```python
from build123d import *

# Parameters (mm, degrees)
F1_DEPTH = 12.7
F2_R     = 15.24
F3_R     = 5.08
F6_DEPTH = 1.27
F9_DEPTH = 1.27


with BuildPart() as f1:
    # F0 (on Front) → F1 (new body)
    with BuildSketch(Plane.XZ):
        with BuildLine():
            ThreePointArc((41.717369, 0.82729), (26.878905, 42.014486), (0, 76.570086))
            ThreePointArc((0, 76.570086), (-26.878905, 42.014486), (-41.717369, 0.82729))
            Line((-41.717369, 0.82729), (-36.542559, 0.82729))
            ThreePointArc((-36.542559, 0.82729), (-23.349687, 37.863578), (0, 69.494744))
            ThreePointArc((0, 69.494744), (23.349687, 37.863578), (36.542559, 0.82729))
            Line((36.542559, 0.82729), (41.717369, 0.82729))
        make_face()
    extrude(amount=F1_DEPTH)

    # F2
    f2_edges = [f1.edges().sort_by_distance(p)[0] for p in [
        (0, -6.35, 76.570086),
    ]]
    fillet(f2_edges, radius=F2_R)

    # F3
    f3_edges = [f1.edges().sort_by_distance(p)[0] for p in [
        (0, -6.35, 69.494744),
    ]]
    fillet(f3_edges, radius=F3_R)

    # F5 (on offset) → F6 (join, symmetric)
    with BuildSketch(Plane.YZ.offset(37.338)):
        with BuildLine():
            Line((-3.302, 0.82729), (-9.398, 0.82729))
            ThreePointArc((-9.398, 0.82729), (-12.734035, -9.091947), (-9.893086, -19.164158))
            Line((-9.893086, -19.164158), (-3.797086, -19.164158))
            ThreePointArc((-3.797086, -19.164158), (-0.461051, -9.24492), (-3.302, 0.82729))
        make_face()
    extrude(amount=F6_DEPTH, both=True)

    # F8 (on offset) → F9 (join, symmetric)
    with BuildSketch(Plane.YZ.offset(-37.338)):
        with BuildLine():
            Line((-3.302, 0.82729), (-9.398, 0.82729))
            ThreePointArc((-9.398, 0.82729), (-12.734035, -9.091947), (-9.893086, -19.164158))
            Line((-9.893086, -19.164158), (-3.797086, -19.164158))
            ThreePointArc((-3.797086, -19.164158), (-0.461051, -9.24492), (-3.302, 0.82729))
        make_face()
    extrude(amount=F9_DEPTH, both=True)


solid = f1.part
```
CAD build for the part. Positions are in the model's coordinates, mm. A direction names the side the tool comes from. Round coordinates to 2 decimals unless told otherwise and drop trailing zeros. Order: outer loops, then holes, each group sorted by start corner. A loop starts at its lowest first (then second) coordinate and runs counter-clockwise, first axis right, second up. Notation, with made-up numbers: (-30, -26.75) - (29, -26.75) arc R30 cw to (29, -4.75) - close; hole circle Ø10 at (81, 19). An arc over 180 degrees is marked (long way). Use CSV: the item, a comma, the result in double quotes. Start each with the question number.
1) Tool access for faces 1 (the flat face through (-36.068, -7, -9)), 2 (the cylindrical face through (-30.54, -6.26, 34.89)), 3 (the flat face through (-38.608, -7, -9)): list every direction of +Z, -Z, +X, -X, +Y, -Y with a clear straight run to the whole face (end or side of a thin tool).
2) Saw through at A-A (z = -10). List the corners of the cut face in (x, y), and give its area (3 significant figures).
3) Saw through at B-B (z = 55). List the corners of the cut face in (x, y), and give its area (3 significant figures).
4) Two-plate mould, pull along Z, no slides. Class faces 4 (the flat face through (38.608, -7, -9)), 5 (the flat face through (40, -6, 0.827)), 6 (the flat face through (37, -7, -19.164)): pulls with the +Z half, pulls with the -Z half, needs draft (parallel to the pull), parting line crosses it, or undercut.
5) Wall check: L1, parallel to X at y = -1.25, z = -13.5; L2, parallel to X at y = -1.5, z = 48.5; L3, parallel to Z at x = -13, y = -2.5. Give the ranges that are in metal, low to high. Write a range as [from, to].
6) Saw through at C-C (x = -17). List the corners of the cut face in (y, z), and give its area (3 significant figures).
7) Pin check, flat tips, straight feed: pin 1 Ø2 at (y, z) = (-9.5, 15.5) entering from -X; pin 2 Ø4 at (y, z) = (-8, 16) entering from +X; pin 3 Ø6 at (y, z) = (-5.5, 26.5) entering from -X. Stop position of each tip, or through.
Values follow:
1,face 1,"-Z, +Y, -Y"
1,face 2,"+Z, -X, +Y, -Y"
1,face 3,"-Z, -X, +Y, -Y"
2,outline,"(-38.61, -12.73) - (-36.07, -12.73) - (-36.07, -0.5) - (-38.61, -0.5) - close; (36.07, -12.73) - (38.61, -12.73) - (38.61, -0.5) - (36.07, -0.5) - close"
2,area,"62.2 mm2"
3,outline,"(-18.77, -12.7) - (-12.5, -12.7) - (-12.5, 0) - (-18.77, 0) - close; (12.5, -12.7) - (18.77, -12.7) - (18.77, 0) - (12.5, 0) - close"
3,area,"159 mm2"
4,face 4,"needs draft"
4,face 5,"undercut"
4,face 6,"pulls with the -Z half"
5,L1,"x = [-38.61, -36.07], [36.07, 38.61]"
5,L2,"x = [-23.08, -17.04], [17.04, 23.08]"
5,L3,"z = [54.32, 62.62]"
6,outline,"(-12.7, 48.57) - (0, 48.57) - (0, 57.45) - (-12.7, 57.45) - close"
6,area,"113 mm2"
7,pin 1,"stops at x = -38.39"
7,pin 2,"stops at x = 38.54"
7,pin 3,"stops at x = -35.38"
